Input: part model. Units: mm. Frame: model coordinates. Face numbers are marked on the shaded views. Give positions to 0.01 mm unless a question says otherwise; leave off trailing zeros. Write each loop counter-clockwise with the first axis right and the second up, starting at its lowest first coordinate (ties: lowest second). Pieces come first, ordered by that corner, then holes.
```python
from build123d import *

# Parameters (mm, degrees)
SKETCH1_W                 = 96
SKETCH1_H                 = 96
BOSS_EXTRUDE1_DEPTH       = 8
SKETCH2_W                 = 92
SKETCH2_H                 = 92
COMPONENT_PLATFORM_DEPTH  = 6
CABLE_SLOTS_DEPTH         = 6
SKETCH4_R                 = 7.75
CENTER_MASS_CUT_DEPTH     = 6
INNER_CORNER_FILLETS_R    = 3
SKETCH10_W                = 12
SKETCH10_H                = 10
MOTOR_CUTOUT_DEPTH        = 2
FILLET1_R                 = 3
M3X0_5_TAPPED_HOLE1_D     = 2.5
M3X0_5_TAPPED_HOLE1_DEPTH = 2
F_3_0MM_DOWEL_HOLE1_D     = 3
F_3_0MM_DOWEL_HOLE1_DEPTH = 2
F_3_0MM_DOWEL_HOLE2_D     = 3
F_3_0MM_DOWEL_HOLE2_DEPTH = 2
F_2_0MM_DOWEL_HOLE1_D     = 2
F_2_0MM_DOWEL_HOLE1_DEPTH = 2
F_4_0MM_DOWEL_HOLE1_D     = 4
F_4_0MM_DOWEL_HOLE1_DEPTH = 2
F_3_0MM_DOWEL_HOLE3_D     = 3
F_3_0MM_DOWEL_HOLE3_DEPTH = 2
SKETCH34_OUTSIDE_W        = 125.2
SKETCH34_OUTSIDE_H        = 125.2
SKETCH34_OUTSIDE_W_2      = 95
SKETCH34_OUTSIDE_H_2      = 95
CUT_EXTRUDE1_DEPTH        = 10


with BuildPart() as part:
    # Sketch1 → Boss-Extrude1 (new body)
    with BuildSketch(Plane.XY):
        Rectangle(SKETCH1_W, SKETCH1_H)
    extrude(amount=BOSS_EXTRUDE1_DEPTH)

    # Sketch2 → Component Platform (cut)
    with BuildSketch(Plane.XY.offset(8)):
        Rectangle(SKETCH2_W, SKETCH2_H)
    extrude(amount=-COMPONENT_PLATFORM_DEPTH, mode=Mode.SUBTRACT)

    # Sketch3 → Cable Slots (cut, symmetric)
    with BuildSketch(Plane.XY.offset(2)):
        with BuildLine():
            Line((-33.878679656, -25.121320344), (-28.878679656, -20.121320344))
            ThreePointArc((-28.878679656, -20.121320344), (-28.228361402, -19.148050297), (-28, -18))
            Line((-28, -18), (-28, 18))
            ThreePointArc((-28, 18), (-28.228361402, 19.148050297), (-28.878679656, 20.121320344))
            Line((-28.878679656, 20.121320344), (-33.878679656, 25.121320344))
            ThreePointArc((-33.878679656, 25.121320344), (-34.851949703, 25.771638598), (-36, 26))
            Line((-36, 26), (-48, 26))
            Line((-48, 26), (-48, -26))
            Line((-48, -26), (-36, -26))
            ThreePointArc((-36, -26), (-34.851949703, -25.771638598), (-33.878679656, -25.121320344))
        make_face()
        with BuildLine():
            Line((48, -26), (48, 26))
            Line((48, 26), (36, 26))
            ThreePointArc((36, 26), (34.851949703, 25.771638598), (33.878679656, 25.121320344))
            Line((33.878679656, 25.121320344), (28.878679656, 20.121320344))
            ThreePointArc((28.878679656, 20.121320344), (28.228361402, 19.148050297), (28, 18))
            Line((28, 18), (28, -18))
            ThreePointArc((28, -18), (28.228361402, -19.148050297), (28.878679656, -20.121320344))
            Line((28.878679656, -20.121320344), (33.878679656, -25.121320344))
            ThreePointArc((33.878679656, -25.121320344), (34.851949703, -25.771638598), (36, -26))
            Line((36, -26), (48, -26))
        make_face()
    extrude(amount=CABLE_SLOTS_DEPTH, both=True, mode=Mode.SUBTRACT)

    # Sketch4 → Center Mass Cut (cut)
    with BuildSketch(Plane.XY.offset(2)):
        Circle(SKETCH4_R)
    extrude(amount=-CENTER_MASS_CUT_DEPTH, mode=Mode.SUBTRACT)

    # Inner Corner Fillets
    inner_corner_fillets_edges = [part.edges().sort_by_distance(p)[0] for p in [
        (-46, -46, 5),
        (-46, 46, 5),
        (46, 46, 5),
        (46, -46, 5),
    ]]
    fillet(inner_corner_fillets_edges, radius=INNER_CORNER_FILLETS_R)

    # Sketch10 → Motor Cutout (cut)
    with BuildSketch(Plane.XY.offset(2)):
        with Locations((6, 0)):
            Rectangle(SKETCH10_W, SKETCH10_H)
    extrude(amount=-MOTOR_CUTOUT_DEPTH, mode=Mode.SUBTRACT)

    # Fillet1
    fillet1_edges = [part.edges().sort_by_distance(p)[0] for p in [
        (12, -5, 1),
        (12, 5, 1),
    ]]
    fillet(fillet1_edges, radius=FILLET1_R)

    # M3x0.5 Tapped Hole1
    with Locations(Plane(origin=(48, 0, 0), x_dir=(0, 0, -1), z_dir=(1, 0, 0))):
        with Locations((-5, -35), (-5, 35)):
            Hole(M3X0_5_TAPPED_HOLE1_D / 2, depth=M3X0_5_TAPPED_HOLE1_DEPTH)

    # Ø3.0mm Dowel Hole1
    with Locations(Plane(origin=(0, 48, 0), x_dir=(1, 0, 0), z_dir=(0, 1, 0))):
        with Locations((35, -5), (-35, -5)):
            f_3_0mm_dowel_hole1 = Hole(F_3_0MM_DOWEL_HOLE1_D / 2, depth=F_3_0MM_DOWEL_HOLE1_DEPTH)

    # Mirror2: Ø3.0mm Dowel Hole1 across plane
    add(f_3_0mm_dowel_hole1.mirror(Plane(origin=(0, 0, 0), x_dir=(0, 0, 1), z_dir=(0, -1, 0))), mode=Mode.SUBTRACT)

    # Ø3.0mm Dowel Hole2
    with Locations(Plane.XY.offset(2)):
        with Locations((-26.5, -26.5), (26.5, -26.5), (26.5, 26.5), (-26.5, 26.5)):
            Hole(F_3_0MM_DOWEL_HOLE2_D / 2, depth=F_3_0MM_DOWEL_HOLE2_DEPTH)

    # Ø2.0mm Dowel Hole1
    with Locations(Plane.XY.offset(2)):
        with Locations((6.72, -6.72), (0, -10), (-6.72, -6.72), (-10, 0), (-6.72, 6.72), (0, 10), (6.72, 6.72)):
            Hole(F_2_0MM_DOWEL_HOLE1_D / 2, depth=F_2_0MM_DOWEL_HOLE1_DEPTH)

    # Ø4.0mm Dowel Hole1
    with Locations(Plane.XY.offset(2)):
        with Locations((-3.74, -20.47), (11.5, -38.25)):
            Hole(F_4_0MM_DOWEL_HOLE1_D / 2, depth=F_4_0MM_DOWEL_HOLE1_DEPTH)

    # Ø3.0mm Dowel Hole3
    with Locations(Plane(origin=(-48, 35, 5), x_dir=(0, 0, -1), z_dir=(-1, 0, 0))):
        with Locations((0, 0), (0, 70)):
            Hole(F_3_0MM_DOWEL_HOLE3_D / 2, depth=F_3_0MM_DOWEL_HOLE3_DEPTH)

    # Sketch34 outside → Cut-Extrude1 (cut)
    with BuildSketch(Plane(origin=(0, 0, 0), x_dir=(-1, 0, 0), z_dir=(0, 0, -1))):
        Rectangle(SKETCH34_OUTSIDE_W, SKETCH34_OUTSIDE_H)
        Rectangle(SKETCH34_OUTSIDE_W_2, SKETCH34_OUTSIDE_H_2, mode=Mode.SUBTRACT)
    extrude(amount=-CUT_EXTRUDE1_DEPTH, mode=Mode.SUBTRACT)


solid = part.part
```
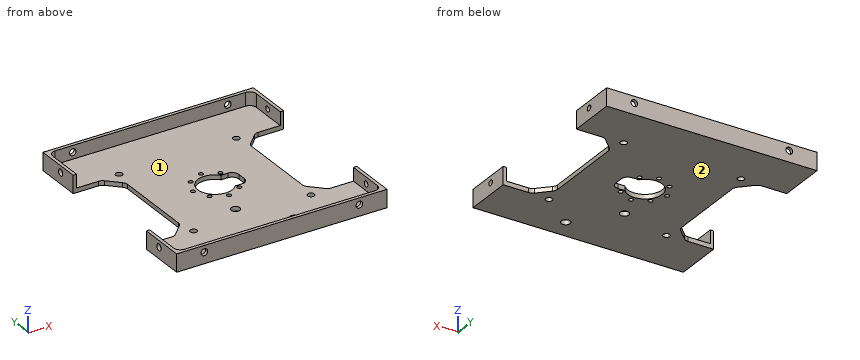
Item 1: Section A-A (y = 35). Return loops of the section in (x, z), and give its area (3 significant figures).
Item 2: Pin query (flat end, axial travel): pin 1 (1.6 mm diameter, centred on y = -4.5, z = 1, fed in from +X); pin 2 (8 mm diameter, centred on x = 17, y = 25.5, fed in from +Z). Return the tip coordinate at first contact, or that it passes through.
Item 3: Mould query, pull axis X, two halves, no side actions, for the marked faces 1 and 2. Classes: +X half, -X half, draft (parallel to the pull), parting line (faces both ways), or undercut.
Item 4: Section D-D (x = -31.5). Return loops of the section in (y, z), and give its area (3 significant figures).
Item 5: Section C-C (x = -3.74). Return loops of the section in (y, z).
Item 6: Section B-B (y = -38.25). Return loops of the section in (x, z).
Item 7: Ray query, line 1 (X direction, y = -46.9, z = 5); line 2 (Y direction, x = 26.5, z = 0.85); line 3 (Y direction, x = -47, z = 5). Return the intervals inside material, ascending.
Solved:
1. outline: (-47.5, 0) - (47.5, 0) - (47.5, 3.75) - (46, 3.75) - (46, 2) - (-46, 2) - (-46, 3.5) - (-47.5, 3.5) - close; (-47.5, 6.5) - (-46, 6.5) - (-46, 8) - (-47.5, 8) - close; (46, 6.25) - (47.5, 6.25) - (47.5, 8) - (46, 8) - close
1. area: 200 mm2
2. pin 1: stops at x = 28
2. pin 2: stops at z = 2
3. face 1: undercut
3. face 2: draft
4. outline: (-47.5, 0) - (-22.74, 0) - (-22.74, 2) - (-46, 2) - (-46, 8) - (-47.5, 8) - close; (22.74, 0) - (47.5, 0) - (47.5, 8) - (46, 8) - (46, 2) - (22.74, 2) - close
4. area: 117 mm2
5. outline: (-47.5, 0) - (-22.47, 0) - (-22.47, 2) - (-46, 2) - (-46, 8) - (-47.5, 8) - close; (-18.47, 0) - (-6.79, 0) - (-6.79, 2) - (-18.47, 2) - close; (6.79, 0) - (47.5, 0) - (47.5, 8) - (46, 8) - (46, 2) - (6.79, 2) - close
6. outline: (-47.5, 0) - (9.5, 0) - (9.5, 2) - (-46, 2) - (-46, 8) - (-47.5, 8) - close; (13.5, 0) - (47.5, 0) - (47.5, 8) - (46, 8) - (46, 2) - (13.5, 2) - close
7. line 1: x = -47.5 to -36.5, -33.5 to 33.5, 36.5 to 47.5
7. line 2: y = -47.5 to -28, -25 to 25, 28 to 47.5
7. line 3: y = -47.5 to -36.5, -33.5 to -26, 26 to 33.5, 36.5 to 47.5
